The listing builds one solid part. Answer for the finished solid, in the listing's coordinates (mm). Face numbers are marked on the shaded views. A direction names the side the tool comes from. Round coordinates to 2 decimals unless told otherwise and drop trailing zeros. Order: outer loops, then holes, each group sorted by start corner. A loop starts at its lowest first (then second) coordinate and runs counter-clockwise, first axis right, second up. Notation, with made-up numbers: M 53,21.5 L 74,21.5 A29 cw 74,54.5 Z; hole C 76,62 d5. An arc over 180 degrees is marked long. Put each result on its own line as item: value. Start each with the question number.
1. The part is cut by section A-A (x = 0). Give the vertices of the cut face in (y, z), then the cut area to 3 significant figures.
2. Which of the six approach directions +Z, -Z, +X, -X, +Y, -Y give full straight-line access (tool end or side, diameter ignored) to the marked faces 1 and 2?
3. Each of these flat-tipped pins is pushed along its axis until it touches: pin 1 Ø8 at (x, y) = (11.5, -18) entering from +Z; pin 2 Ø1.5 at (x, z) = (-18, 3) entering from +Y; pin 3 Ø2 at (x, z) = (-13.5, 3.5) entering from -Y; pin 4 Ø4 at (y, z) = (-2.5, 0) entering from +X. Where does it stop, or does it pass through?
4. The part is cut by section D-D (z = -2.5). Give the vertices of the cut face in (x, y).
5. Consider line 1 (Y direction, x = 0, z = -3); line 2 (Y direction, x = 0, z = 6.25); line 3 (Z direction, x = 3.5, y = 18.5). Determine where each line is inside the solid, lowest interval first.
6. The part is cut by section C-C (z = 5). Give the vertices of the cut face in (x, y), then the cut area to 3 significant figures.
7. The mould has two halves that part along X. Classify the marked faces 3, 4 and 5: +X half, -X half, draft (parallel to the pull), parting line (faces both ways), or undercut.
from build123d import *

# Parameters (mm, degrees)
SKETCH1_R           = 23
BOSS_EXTRUDE1_DEPTH = 11.4
SKETCH2_R           = 20.5
CUT_EXTRUDE1_DEPTH  = 8
SKETCH3_R           = 16.99
BOSS_EXTRUDE2_DEPTH = 7.8
SKETCH4_R           = 15
CUT_EXTRUDE2_DEPTH  = 34.496268449
FILLET1_R           = 1
FILLET3_R           = 1
FILLET4_R           = 1


with BuildPart() as part:
    # Sketch1 → Boss-Extrude1 (new body)
    with BuildSketch(Plane.XY):
        Circle(SKETCH1_R)
    extrude(amount=BOSS_EXTRUDE1_DEPTH)

    # Sketch2 → Cut-Extrude1 (cut)
    with BuildSketch(Plane.XY.offset(11.4)):
        Circle(SKETCH2_R)
    extrude(amount=-CUT_EXTRUDE1_DEPTH, mode=Mode.SUBTRACT)

    # Sketch3 → Boss-Extrude2 (add)
    with BuildSketch(Plane.XY.offset(3.4)):
        Circle(SKETCH3_R)
    extrude(amount=-BOSS_EXTRUDE2_DEPTH)

    # Sketch4 → Cut-Extrude2 (cut, through all)
    with BuildSketch(Plane.XY.offset(3.4)):
        Circle(SKETCH4_R)
    extrude(amount=-CUT_EXTRUDE2_DEPTH, mode=Mode.SUBTRACT)

    # Fillet1
    fillet1_edges = [part.edges().sort_by_distance(p)[0] for p in [
        (-15, 0, 3.4),
    ]]
    fillet(fillet1_edges, radius=FILLET1_R)

    # Fillet3
    fillet3_edges = [part.edges().sort_by_distance(p)[0] for p in [
        (-16.99, 0, -4.4),
        (-23, 0, 11.4),
        (-20.5, 0, 11.4),
    ]]
    fillet(fillet3_edges, radius=FILLET3_R)

    # Fillet4
    fillet4_edges = [part.edges().sort_by_distance(p)[0] for p in [
        (-23, 0, 0),
    ]]
    fillet(fillet4_edges, radius=FILLET4_R)


solid = part.part
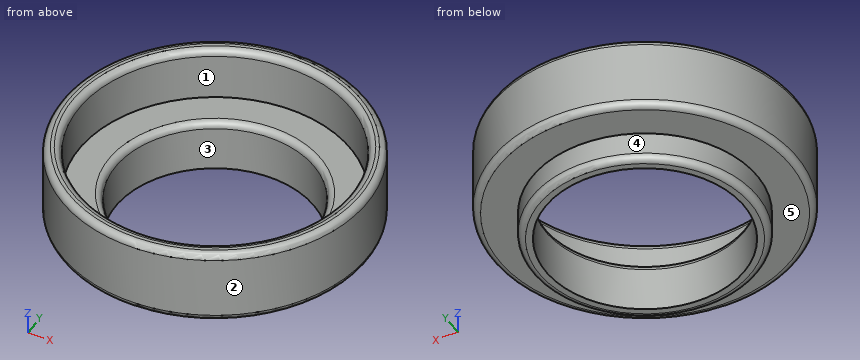
Resolved:
1. outline: M -23,1 A1 ccw -22,0 L -16.99,0 L -16.99,-3.4 A1 ccw -15.99,-4.4 L -15,-4.4 L -15,2.4 A1 ccw -16,3.4 L -20.5,3.4 L -20.5,10.4 A1 ccw -21.5,11.4 L -22,11.4 A1 ccw -23,10.4 Z; M 15,-4.4 L 15.99,-4.4 A1 ccw 16.99,-3.4 L 16.99,0 L 22,0 A1 ccw 23,1 L 23,10.4 A1 ccw 22,11.4 L 21.5,11.4 A1 ccw 20.5,10.4 L 20.5,3.4 L 16,3.4 A1 ccw 15,2.4 Z
1. area: 110 mm2
2. face 1: +Z
2. face 2: +Z, -Z
3. pin 1: z = 11.4
3. pin 2: y = 15.21
3. pin 3: y = -19.31
3. pin 4: x = 22.99
4. outline: C 0,0 d33.98; hole C 0,0 d30
5. line 1: -16.99 to -15, 15 to 16.99
5. line 2: -23 to -20.5, 20.5 to 23
5. line 3: 0 to 3.4
6. outline: C 0,0 d46; hole C 0,0 d41
6. area: 342 mm2
7. face 3: undercut
7. face 4: parting line
7. face 5: draft
